CAD build for the part. Positions are in the model's coordinates, mm. A direction names the side the tool comes from. Give positions to 0.01 mm unless a question says otherwise; leave off trailing zeros. Write each loop counter-clockwise with the first axis right and the second up, starting at its lowest first coordinate (ties: lowest second). Pieces come first, ordered by that corner, then holes. Notation, with made-up numbers: (-29, 19) - (-14, 19) arc R15 cw to (-14, 34) - close; hole circle Ø8 at (79, 50). An arc over 180 degrees is marked (long way). Put each result on its own line as item: value. Start each with the question number.
1. Cut at D-D on z = 7.5. List the corners of the cut face in (x, y), and give its area (3 significant figures).
2. Cut at B-B on x = -11. List the corners of the cut face in (y, z), and give its area (3 significant figures).
3. Drop flat-ended pins along their axis: pin 1 (6 mm diameter, centred on x = 10.5, z = 16, fed in from -Y); pin 2 (3 mm diameter, centred on y = -6.5, z = 20.5, fed in from +X); pin 3 (12 mm diameter, centred on x = 3.5, z = 27.5, fed in from -Y). Give the stop position or say it passes through.
4. Cut at C-C on z = 23. List the corners of the cut face in (x, y).
5. Cut at A-A on y = -18.75. List the corners of the cut face in (x, z).
6. Mould opens along X. For faces 1 (the flat face through (-37, -25.4, 17)), 2 (the cylindrical face through (-42.046, -12.522, 33.13)), 3 (the cylindrical face through (-19.267, -13.228, 11.133)) say: +X half, -X half, draft (parallel to the pull), parting line (faces both ways), or undercut.
7. Tool access for faces 4 (the flat face through (-23, -13, 4.694)), 5 (the flat face through (-38.266, -13, 22)): list every direction of +Z, -Z, +X, -X, +Y, -Y with a clear straight run to the whole face (end or side of a thin tool).
8. Wall check: line 1 (Y direction, x = -1, z = 13); line 2 (X direction, y = -13, z = 8.5); line 3 (Z direction, x = 7.5, y = -5.25). Give the ranges that are in metal, low to high.
from build123d import *

# Parameters (mm, degrees)
F1_DEPTH = 25.4
F4_DEPTH = 25.4
F5_R     = 6.35
F6_DEPTH = 25.4
F8_DEPTH = 25.4


with BuildPart() as f1:
    # F0 (on Front) → F1 (new body)
    with BuildSketch(Plane.XZ):
        with BuildLine():
            Line((-48.741896, 36.444197), (-53.308046, 36.444197))
            ThreePointArc((-53.308046, 36.444197), (-59.769484, 33.341808), (-63.66557, 27.325537))
            Line((-63.66557, 27.325537), (-63.66557, 4.694197))
            Line((-63.66557, 4.694197), (18.88443, 4.694197))
            Line((18.88443, 4.694197), (18.88443, 17.394197))
            Line((18.88443, 17.394197), (-38.26557, 17.394197))
            Line((-38.26557, 17.394197), (-38.26557, 26.919197))
            ThreePointArc((-38.26557, 26.919197), (-42.1227, 33.200663), (-48.741896, 36.444197))
        make_face()
    extrude(amount=F1_DEPTH)

    # F3 (on face) → F4 (cut)
    with BuildSketch(Plane.XY.offset(17.394197)):
        with BuildLine():
            ThreePointArc((6.368123, 0), (18.857612, -12.305201), (7.198642, -25.4))
            Line((7.198642, -25.4), (18.88443, -25.4))
            Line((18.88443, -25.4), (18.88443, 0))
            Line((18.88443, 0), (6.368123, 0))
        make_face()
    extrude(amount=-F4_DEPTH, mode=Mode.SUBTRACT)

    # F5 (on face) → F6 (cut)
    with BuildSketch(Plane.XZ.offset(25.4)):
        with Locations((-51.028371, 23.744197)):
            Circle(F5_R)
    extrude(amount=-F6_DEPTH, mode=Mode.SUBTRACT)

    # F7 (on face) → F8 (cut)
    with BuildSketch(Plane.XY.offset(17.394197)):
        with BuildLine():
            ThreePointArc((-0.085432, -19.59818), (4.352802, -17.71039), (6.18443, -13.248686))
            ThreePointArc((6.18443, -13.248686), (4.295666, -8.729851), (-0.247025, -6.899208))
            ThreePointArc((-0.247025, -6.899208), (-6.515056, -13.329482), (-0.085432, -19.59818))
        make_face()
        with BuildLine():
            ThreePointArc((-0.085432, -19.59818), (-6.515056, -13.329482), (-0.247025, -6.899208))
            Line((-0.247025, -6.899208), (-12.835866, -7.060705))
            ThreePointArc((-12.835866, -7.060705), (-8.39968, -8.949577), (-6.569161, -13.410158))
            ThreePointArc((-6.569161, -13.410158), (-8.372724, -17.843262), (-12.758896, -19.758136))
            Line((-12.758896, -19.758136), (-0.085432, -19.59818))
        make_face()
        with BuildLine():
            ThreePointArc((-6.569161, -13.410158), (-8.39968, -8.949577), (-12.835866, -7.060705))
            ThreePointArc((-12.835866, -7.060705), (-19.269025, -13.36851), (-12.919161, -19.760158))
            Line((-12.919161, -19.760158), (-12.758896, -19.758136))
            ThreePointArc((-12.758896, -19.758136), (-8.372724, -17.843262), (-6.569161, -13.410158))
        make_face()
        with BuildLine():
            ThreePointArc((-12.919161, -19.760158), (-12.839022, -19.759653), (-12.758896, -19.758136))
            Line((-12.758896, -19.758136), (-12.919161, -19.760158))
        make_face()
    extrude(amount=-F8_DEPTH, mode=Mode.SUBTRACT)


solid = f1.part
Report:
1. outline: (-63.67, -25.4) - (7.2, -25.4) arc R12.72 ccw to (6.37, 0) - (-63.67, 0) - close; hole (-12.92, -19.76) arc R6.35 ccw to (-12.76, -19.76) - (-0.09, -19.6) arc R6.35 ccw to (6.18, -13.25) arc R6.35 ccw to (-0.25, -6.9) - (-12.84, -7.06) arc R6.35 ccw (long way) to start
1. area: 1,740 mm²
2. outline: (-25.4, 4.69) - (-19.74, 4.69) - (-19.74, 17.39) - (-25.4, 17.39) - close; (-7.04, 4.69) - (0, 4.69) - (0, 17.39) - (-7.04, 17.39) - close
2. area: 161 mm²
3. pin 1: stops at y = -25.37
3. pin 2: stops at x = -38.27
3. pin 3: passes through
4. outline: (-63.67, -25.4) - (-57.33, -25.4) - (-57.33, 0) - (-63.67, 0) - close; (-44.72, -25.4) - (-38.27, -25.4) - (-38.27, 0) - (-44.72, 0) - close
5. outline: (-63.67, 4.69) - (-16.36, 4.69) - (-16.36, 17.39) - (-38.27, 17.39) - (-38.27, 26.92) arc R13.23 ccw to (-48.74, 36.44) - (-53.31, 36.44) arc R13.23 ccw to (-63.67, 27.33) - close; (3.01, 4.69) - (17.35, 4.69) - (17.35, 17.39) - (3.01, 17.39) - close; hole circle Ø12.7 at (-51.03, 23.74)
6. face 1: draft
6. face 2: +X half
6. face 3: undercut
7. face 4: -Z, +X, -X, +Y, -Y
7. face 5: +Z, +X, +Y, -Y
8. line 1: y = -25.4 to -19.61, -6.91 to 0
8. line 2: x = -63.67 to -19.26, 6.18 to 18.86
8. line 3: z = 4.69 to 17.39
